Read the model definition and answer for the solid it produces. Units are mm, in the model's axes. A direction names the side the tool comes from. Coordinates: 2 decimals unless noted, no trailing zeros. Order: outer loops, then holes, each group sorted by start corner. A loop starts at its lowest first (then second) coordinate and runs counter-clockwise, first axis right, second up. Notation, with made-up numbers: (82, -10) -> (139, -10) arc R33 ccw to (139, 24) -> close; hole circle Ø8 at (83, 6). An arc over 180 degrees is marked (long way). Answer as a JSON object with one key per item and string values. Group by question number.
1) A tool of negligible diameter and unlimited length cuts with its end or side. For faces 1 (the flat face through (4.6, 36.42, 0.4)), 2 (the flat face through (3, 14, 0.8)), from which of +Z, -Z, +X, -X, +Y, -Y can it reach the whole face along a straight path? Write none if from no direction.
2) Section A-A on y = 15 is taken. Determine the outline of the cut face in (x, z), and give its area (3 significant figures).
3) Determine the mould class of faces 3 (the flat face through (6, 14, 0.8)), 4 (the flat face through (4.6, 0, 0.4)), 5 (the flat face through (0, 18, 0.4)) for opening direction Y: released by +Y, released by -Y, zero draft, split by the parting line, or undercut.
4) Given pin 1 (0.7 mm diameter, centred on x = 5.5, y = 13, fed in from +Z), flat-ended and moving along its own axis, determine where the tip first touches the part or whether it passes through.
from build123d import *

# Parameters (mm, degrees)
SKETCH_W     = 9.4
SKETCH_H     = 36.42
SKETCH_W_2   = 0.1
SKETCH_H_2   = 5
PAD_DEPTH    = 0.9
SKETCH001_W  = 5
SKETCH001_H  = 5
POCKET_DEPTH = 0.1


with BuildPart() as part:
    # Sketch → Pad (new body)
    with BuildSketch(Plane.XY):
        with Locations((4.7, 18.21)):
            Rectangle(SKETCH_W, SKETCH_H)
        with Locations((4.7, 13.9)):
            Rectangle(SKETCH_W_2, SKETCH_H_2, mode=Mode.SUBTRACT)
    extrude(amount=PAD_DEPTH)

    # Sketch001 (on Face10 of Pad) → Pocket (cut)
    with BuildSketch(Plane.XY.offset(0.9)):
        with Locations((4.7, 13.9)):
            Rectangle(SKETCH001_W, SKETCH001_H)
    extrude(amount=-POCKET_DEPTH, mode=Mode.SUBTRACT)


solid = part.part
Worked answers:
{
 "1": {"face 1": "+Z, -Z, +X, -X, +Y", "face 2": "+Z"},
 "2": {"outline": "(0, 0) -> (4.65, 0) -> (4.65, 0.8) -> (2.2, 0.8) -> (2.2, 0.9) -> (0, 0.9) -> close; (4.75, 0) -> (9.4, 0) -> (9.4, 0.9) -> (7.2, 0.9) -> (7.2, 0.8) -> (4.75, 0.8) -> close", "area": "7.88 mm²"},
 "3": {"face 3": "undercut", "face 4": "released by -Y", "face 5": "zero draft"},
 "4": {"pin 1": "stops at z = 0.8"}
}
